from build123d import *

# Parameters (mm, degrees)
F0_W     = 20.271596
F0_H     = 5.08
F3_D     = 9.525
F3_DEPTH = 50.8


with BuildPart() as f1:
    # F0 (on Front) → F1 (revolve)
    with BuildSketch(Plane.XZ):
        with Locations((-10.135798, 5.08)):
            Rectangle(F0_W, F0_H)
        Polygon((-20.271596, 7.62), (0, 7.62), (0, 10.16), (-25.4, 10.16), (-25.4, 7.62), align=None)
        Polygon((-25.4, 0), (0, 0), (0, 2.54), (-20.271596, 2.54), (-25.4, 2.54), align=None)
    revolve(axis=Axis((0, 0, 5.08), (0, 0, 1)))

    # F3
    with Locations(Plane.XY.offset(10.16)):
        with Locations((0, 0)):
            Hole(F3_D / 2, depth=F3_DEPTH)


solid = f1.part
Can you work these out from the model? Positions are in its coordinate system, mm. A direction names the side the tool comes from. Give positions to 0.01 mm unless a question says otherwise; leave off trailing zeros. Loops run counter-clockwise (first coordinate to the right, second up) from the corner with the lowest first, then second, coordinate; pieces in that order, holes last. Notation, with made-up numbers: M 31.5,79.5 L 90.5,79.5 A25 ccw 90.5,100.5 Z; hole C -21,-14.75 d9. An arc over 180 degrees is marked long. One line per item, written item: value. Start each with the question number.
1) If we section it at A-A, the plane y = 0: Write out the boundary of the cut face in (x, z).
2) If I drill on line 1 (Y direction, x = 0, z = 4.25); line 2 (Z direction, x = -21, y = 3); line 3 (Y direction, x = 4, z = 1), over which ranges is the centre line in solid material (lowest first)? Write a range as [from, to].
3) If we section it at C-C, the plane z = 8.75: Write out the boundary of the cut face in (x, y) (1 decimal).
4) Thinking about a two-plate mould opening in Z: for faces 3 (the face through (17.1, 11.2, 7.62)), 4 (the face through (5.506, 24.796, 8.872)), 5 (the face through (5, 0, 10.16)), 6 (the face through (-5, 0, 0)), which applies, +Z half, -Z half, draft (parallel to the pull), parting line (faces both ways), or undercut?
5) I'm going to push flat-ended pins straight in: pin 1 (5.5 mm diameter, centred on x = 0, y = 0, fed in from +Z); pin 2 (3 mm diameter, centred on x = -16, z = 7.5, fed in from +Y). Where does each tip first touch, or does it pass through?
6) If we section it at D-D, the plane y = 11: Write out the boundary of the cut face in (x, z).
7) On a 3-axis mill with a long thin cutter (end or side, diameter ignored), from which of +Z, -Z, +X, -X, +Y, -Y can I reach the whole of each face in a straight line? I mean faces 1 (the face through (-17.1, 11.2, 2.54)), 2 (the face through (3.78, -2.9, 5.01)). Say none if no direction works.
Completed:
1. outline: M -25.4,0 L -4.76,0 L -4.76,10.16 L -25.4,10.16 L -25.4,7.62 L -20.27,7.62 L -20.27,2.54 L -25.4,2.54 Z; M 4.76,0 L 25.4,0 L 25.4,2.54 L 20.27,2.54 L 20.27,7.62 L 25.4,7.62 L 25.4,10.16 L 4.76,10.16 Z
2. line 1: y = [-20.27, -4.76], [4.76, 20.27]
2. line 2: z = [0, 2.54], [7.62, 10.16]
2. line 3: y = [-25.08, -2.58], [2.58, 25.08]
3. outline: C 0,0 d50.8; hole C 0,0 d9.5
4. face 3: undercut
4. face 4: draft
4. face 5: +Z half
4. face 6: -Z half
5. pin 1: passes through
5. pin 2: stops at y = 20.85
6. outline: M -22.89,0 L 22.89,0 L 22.89,2.54 L 17.03,2.54 L 17.03,7.62 L 22.89,7.62 L 22.89,10.16 L -22.89,10.16 L -22.89,7.62 L -17.03,7.62 L -17.03,2.54 L -22.89,2.54 Z
7. face 1: none
7. face 2: +Z, -Z
